```python
from build123d import *

# Parameters (mm, degrees)
SKETCH1_W           = 60
SKETCH1_H           = 40
BOSS_EXTRUDE1_DEPTH = 3
SKETCH2_R           = 2
CUT_EXTRUDE1_DEPTH  = 3
SKETCH3_R           = 2.5
CUT_EXTRUDE2_DEPTH  = 3


with BuildPart() as part:
    # Sketch1 → Boss-Extrude1 (new body)
    with BuildSketch(Plane(origin=(0, 0, 0), x_dir=(1, 0, 0), z_dir=(0, 1, 0))):
        Rectangle(SKETCH1_W, SKETCH1_H)
    extrude(amount=BOSS_EXTRUDE1_DEPTH)

    # Sketch2 → Cut-Extrude1 (cut)
    with BuildSketch(Plane(origin=(0, 3, 0), x_dir=(1, 0, 0), z_dir=(0, 1, 0))):
        with Locations((-15, 12)):
            Circle(SKETCH2_R)
        with Locations((15, 12)):
            Circle(SKETCH2_R)
        with Locations((15, -12)):
            Circle(SKETCH2_R)
        with Locations((-15, -12)):
            Circle(SKETCH2_R)
    extrude(amount=-CUT_EXTRUDE1_DEPTH, mode=Mode.SUBTRACT)

    # Sketch3 → Cut-Extrude2 (cut)
    with BuildSketch(Plane(origin=(0, 3, 0), x_dir=(1, 0, 0), z_dir=(0, 1, 0))):
        with Locations((-25, 15)):
            Circle(SKETCH3_R)
        with Locations((-25, -15)):
            Circle(SKETCH3_R)
        with Locations((25, 15)):
            Circle(SKETCH3_R)
        with Locations((25, -15)):
            Circle(SKETCH3_R)
    extrude(amount=-CUT_EXTRUDE2_DEPTH, mode=Mode.SUBTRACT)


solid = part.part
```
Build history of the part. All positions in model axes, mm. Coordinates: 2 decimals unless noted, no trailing zeros. Order: outer loops, then holes, each group sorted by start corner. A loop starts at its lowest first (then second) coordinate and runs counter-clockwise, first axis right, second up.
Item 1: Saw through at B-B on y = 0.95. State how many separate pieces and enclosed holes the cut face has, then the cut area to 3 significant figures.
Filled in:
separate pieces: 1
enclosed holes: 8
area: 2,270 mm2
Item 2: Drill centre lines: L1, parallel to Z at x = -15, y = 0.9; L2, parallel to Z at x = 25, y = 1.55; L3, parallel to X at y = 2.4, z = -13. Where is each one in solid material? Low to high.
Filled in:
L1: z = -20 to -14, -10 to 10, 14 to 20
L2: z = -20 to -17.5, -12.5 to 12.5, 17.5 to 20
L3: x = -30 to -26.5, -23.5 to -16.73, -13.27 to 13.27, 16.73 to 23.5, 26.5 to 30
Item 3: Saw through at C-C on x = -25. List the corners of the cut face in (y, z).
Filled in:
outline: (0, -20) - (3, -20) - (3, -17.5) - (0, -17.5) - close; (0, -12.5) - (3, -12.5) - (3, 12.5) - (0, 12.5) - close; (0, 17.5) - (3, 17.5) - (3, 20) - (0, 20) - close
Item 4: Mould opens along X. For faces 1 (the flat face through (-30, 1, 0)), 2 (the cylindrical face through (-15, 2, 10)), 3 (the flat face through (30, 1, 0)), 4 (the flat face through (0, 1, -20)) say: released by +X, released by -X, zero draft, split by the parting line, or undercut.
Filled in:
face 1: released by -X
face 2: undercut
face 3: released by +X
face 4: zero draft
Item 5: Drop a flat-ended pin along its axis: pin 1 Ø5 at (x, z) = (15, -12) entering from +Y. Give the stop position or say it passes through.
Filled in:
pin 1: stops at y = 3
Item 6: Saw through at A-A on x = -15. List the corners of the cut face in (y, z).
Filled in:
outline: (0, -20) - (3, -20) - (3, -14) - (0, -14) - close; (0, -10) - (3, -10) - (3, 10) - (0, 10) - close; (0, 14) - (3, 14) - (3, 20) - (0, 20) - close
